```python
from build123d import *

# Parameters (mm, degrees)
SKETCH1_W                  = 154
SKETCH1_H                  = 125
BOSS_EXTRUDE1_DEPTH        = 1.5
SKETCH2_W                  = 2
SKETCH2_H                  = 5
BOSS_EXTRUDE2_DEPTH        = 5
SKETCH3_W                  = 8
SKETCH3_H                  = 2
BOSS_EXTRUDE3_DEPTH        = 17
SKETCH4_W                  = 2
SKETCH4_H                  = 10.5
BOSS_EXTRUDE4_DEPTH        = 8
CHAMFER1_SIZE              = 2
LPATTERN1_COUNT            = 2
LPATTERN1_PITCH            = 60
CHAMFER1_OF_LPATTERN1_SIZE = 2
SKETCH5_W                  = 5
SKETCH5_H                  = 3
BOSS_EXTRUDE5_DEPTH        = 8
CUT_EXTRUDE1_REACH         = 146.611
SKETCH6_R                  = 1.5
LPATTERN2_COUNT            = 2
LPATTERN2_PITCH            = 125
MIRROR1_START              = -31
MIRROR1_DEPTH              = 8
MIRROR1_START_2            = 29
MIRROR1_2_DEPTH            = 8
MIRROR1_START_3            = 71
MIRROR1_3_OUTLINE_W        = 5
MIRROR1_3_OUTLINE_H        = 5
MIRROR1_3_DEPTH            = 2
MIRROR1_START_4            = 55.5
MIRROR1_4_OUTLINE_W        = 5
MIRROR1_4_OUTLINE_H        = 8
MIRROR1_4_OUTLINE_R        = 1.5
MIRROR1_4_DEPTH            = 3


# Read off the part's stored shape, not the designer's step: Mirror1
with BuildPart() as part:
    # Sketch1 → Boss-Extrude1 (new body)
    with BuildSketch(Plane(origin=(0, 0, 0), x_dir=(1, 0, 0), z_dir=(0, 1, 0))):
        Rectangle(SKETCH1_W, SKETCH1_H)
    extrude(amount=BOSS_EXTRUDE1_DEPTH)

    # Sketch2 → Boss-Extrude2 (add)
    with BuildSketch(Plane(origin=(0, 1.5, 0), x_dir=(1, 0, 0), z_dir=(0, 1, 0))):
        with Locations((72, 56)):
            Rectangle(SKETCH2_W, SKETCH2_H)
    extrude(amount=BOSS_EXTRUDE2_DEPTH)

    # Sketch3 → Boss-Extrude3 (add)
    with BuildSketch(Plane(origin=(0, 1.5, 0), x_dir=(1, 0, 0), z_dir=(0, 1, 0))):
        with Locations((-27, 57.5)):
            Rectangle(SKETCH3_W, SKETCH3_H)
    boss_extrude3 = extrude(amount=BOSS_EXTRUDE3_DEPTH)

    # Sketch4 → Boss-Extrude4 (add)
    with BuildSketch(Plane.ZY.offset(31)):
        with Locations((-59.5, 13.25)):
            Rectangle(SKETCH4_W, SKETCH4_H)
    boss_extrude4 = extrude(amount=-BOSS_EXTRUDE4_DEPTH)

    # Chamfer1
    chamfer1_edges = [part.edges().sort_by_distance(p)[0] for p in [
        (-27, 18.5, -60.5),
        (-27, 8, -60.5),
    ]]
    chamfer(chamfer1_edges, length=CHAMFER1_SIZE - 0.0001)  # a hair under: the kernel refuses the full size

    # LPattern1: Boss-Extrude3, Boss-Extrude4 ×2
    with Locations(*[(i * LPATTERN1_PITCH, 0, 0) for i in range(1, LPATTERN1_COUNT)]):
        add(boss_extrude3)
        add(boss_extrude4)

    # Chamfer1 of LPattern1
    chamfer1_of_lpattern1_edges = [part.edges().sort_by_distance(p)[0] for p in [
        (33, 18.5, -60.5),
        (33, 8, -60.5),
    ]]
    chamfer(chamfer1_of_lpattern1_edges, length=CHAMFER1_OF_LPATTERN1_SIZE - 0.0001)  # a hair under: the kernel refuses the full size

    # Sketch5 → Boss-Extrude5 (add)
    with BuildSketch(Plane(origin=(0, 1.5, 0), x_dir=(1, 0, 0), z_dir=(0, 1, 0))):
        with Locations((67, 57)):
            Rectangle(SKETCH5_W, SKETCH5_H)
    boss_extrude5 = extrude(amount=BOSS_EXTRUDE5_DEPTH)

    # Sketch6 → Cut-Extrude1 (cut, up to next)
    with BuildSketch(Plane(origin=(0, 0, -58.5), x_dir=(-1, 0, 0), z_dir=(0, 0, -1)), mode=Mode.PRIVATE) as cut_extrude1_sk1:
        with Locations((-67, 6.5)):
            Circle(SKETCH6_R)
    cut_extrude1_tool1 = extrude(cut_extrude1_sk1.sketch, amount=-CUT_EXTRUDE1_REACH, mode=Mode.PRIVATE) & part.part
    cut_extrude1 = cut_extrude1_tool1.solids().sort_by_distance((67, 6.5, -58.5))[0]
    add(cut_extrude1, mode=Mode.SUBTRACT)

    # LPattern2: Boss-Extrude5, Cut-Extrude1 ×2
    with Locations(*[(-i * LPATTERN2_PITCH, 0, 0) for i in range(1, LPATTERN2_COUNT)]):
        add(boss_extrude5)
        add(cut_extrude1, mode=Mode.SUBTRACT)

    # Mirror1 outline → Mirror1 (add)
    with BuildSketch(Plane.YZ.offset(MIRROR1_START)):
        Polygon((10, 60.5), (8, 58.5), (1.5, 58.5), (1.5, 56.5), (18.5, 56.5), (18.5, 58.5), (16.5, 60.5), align=None)
    extrude(amount=MIRROR1_DEPTH)

    # Mirror1 2 outline → Mirror1 2 (add)
    with BuildSketch(Plane.YZ.offset(MIRROR1_START_2)):
        Polygon((10, 60.5), (8, 58.5), (1.5, 58.5), (1.5, 56.5), (18.5, 56.5), (18.5, 58.5), (16.5, 60.5), align=None)
    extrude(amount=MIRROR1_2_DEPTH)

    # Mirror1 3 outline → Mirror1 3 (add)
    with BuildSketch(Plane.YZ.offset(MIRROR1_START_3)):
        with Locations((4, 56)):
            Rectangle(MIRROR1_3_OUTLINE_W, MIRROR1_3_OUTLINE_H)
    extrude(amount=MIRROR1_3_DEPTH)

    # Mirror1 4 outline → Mirror1 4 (add)
    # profile 1 of 2: a face of its own
    with BuildSketch(Plane.XY.offset(MIRROR1_START_4)):
        with Locations((67, 5.5)):
            Rectangle(MIRROR1_4_OUTLINE_W, MIRROR1_4_OUTLINE_H)
        with Locations((67, 6.5)):
            Circle(MIRROR1_4_OUTLINE_R, mode=Mode.SUBTRACT)
    # profile 2 of 2: a face of its own
    with BuildSketch(Plane.XY.offset(MIRROR1_START_4)):
        with Locations((-58, 5.5)):
            Rectangle(MIRROR1_4_OUTLINE_W, MIRROR1_4_OUTLINE_H)
        with Locations((-58, 6.5)):
            Circle(MIRROR1_4_OUTLINE_R, mode=Mode.SUBTRACT)
    extrude(amount=MIRROR1_4_DEPTH)


solid = part.part
```
Can you work these out from the model? Positions are in its coordinate system, mm. A direction names the side the tool comes from. Give positions to 0.01 mm unless a question says otherwise; leave off trailing zeros. Loops run counter-clockwise (first coordinate to the right, second up) from the corner with the lowest first, then second, coordinate; pieces in that order, holes last. Notation, with made-up numbers: M 0.5,45.25 L 29.5,45.25 A27 ccw 29.5,77.25 Z; hole C -23,22 d10. An arc over 180 degrees is marked long. Answer in a Markdown table with one row per item.
1. Thinking about a two-plate mould opening in Y: for faces 6 (the flat face through (33, 5, 58.5)), 7 (the flat face through (-1, 0, -1)), 8 (the flat face through (33, 10, 56.5)), which applies, released by +Y, released by -Y, zero draft, split by the parting line, or undercut?
Taken from the geometry:
| item | result |
|---|---|
| face 6 | undercut |
| face 7 | released by -Y |
| face 8 | zero draft |
2. Suppose I cut it at A-A on x = 21.5. Write out the boundary of the cut face in (y, z), plus the area to 4 significant figures.
Taken from the geometry:
| item | result |
|---|---|
| outline | M 0,-62.5 L 1.5,-62.5 L 1.5,62.5 L 0,62.5 Z |
| area | 187.5 mm² |
3. Suppose I cut it at B-B on z = -35. Write out the boundary of the cut face in (x, y), plus the area to 3 significant figures.
Taken from the geometry:
| item | result |
|---|---|
| outline | M -77,0 L 77,0 L 77,1.5 L -77,1.5 Z |
| area | 231 mm² |
4. For pin 1 Ø3.5 at (y, z) = (7, 57.5) entering from +X; pin 2 Ø1.2 at (y, z) = (12.5, 59.5) entering from -X; pin 3 Ø1.6 at (x, z) = (72, 56) entering from +Y, each with a flat end and sliding along its axis, tell me the tip position at first contact or that it passes through.
Taken from the geometry:
| item | result |
|---|---|
| pin 1 | stops at x = 73 |
| pin 2 | stops at x = -31 |
| pin 3 | stops at y = 6.5 |
5. Which directions (+Z, -Z, +X, -X, +Y, -Y) give clear straight access to the entire face, cutting with the end or side of a thin tool? Please do faces 1 (the flat face through (73, 4, -56)), 2 (the flat face through (33, 13, 60.5)), 3 (the flat face through (-58, 4.6, -55.5)), 4 (the flat face through (64.5, 5, -57)), 5 (the flat face through (-27, 13, -60.5)).
Taken from the geometry:
| item | result |
|---|---|
| face 1 | +Z, -Z, +X, +Y |
| face 2 | +Z, +X, -X, +Y |
| face 3 | -X, +Y |
| face 4 | +Z, -Z, +Y |
| face 5 | -Z, +X, -X, +Y |
6. If I drill on line 1 along Y through (x, z) = (67, 56.7); line 2 along Y through (x, z) = (-63, 18); line 3 along X through (y, z) = (4.75, -55), over which ranges is the centre line in solid material (lowest first)?
Taken from the geometry:
| item | result |
|---|---|
| line 1 | y = 0 to 5, 8 to 9.5 |
| line 2 | y = 0 to 1.5 |
| line 3 | x = 71 to 73 |
